Read the model definition and answer for the solid it produces. Units are mm, in the model's axes. Face numbers are marked on the shaded views. A direction names the side the tool comes from. Coordinates: 2 decimals unless noted, no trailing zeros. Loops run counter-clockwise (first coordinate to the right, second up) from the corner with the lowest first, then second, coordinate; pieces in that order, holes last.
Q1. Which of the six approach directions +Z, -Z, +X, -X, +Y, -Y give full straight-line access (tool end or side, diameter ignored) to the marked faces 1 and 2?
Q2. Flat-ended cylindrical pins translate along their axes: P1, Ø1.5, axis at x = 43.5, z = 3.5, coming from the -Y side; P2, Ø1.5, axis at y = 9, z = 2.5, coming from the -X side; P3, Ø2.5, axis at y = -28, z = 3, coming from the +X side; P4, Ø6, axis at x = 80.93, y = -12.5, coming from the +Z side. Find the tip coordinate at first contact, or state that the pin passes through.
Q3. Section D-D (x = 40) is taken. Give the vertices of the cut face in (y, z).
Q4. Straight lines are drawn through the part: line 1 (X direction, y = -26, z = 3.4); line 2 (X direction, y = -12.5, z = 0.9); line 3 (Y direction, x = 57, z = 3.6). For each, find the intervals that lie inside material, in ascending order.
Q5. Section C-C (x = -19) is taken. Give the vertices of the cut face in (y, z), then the cut area to 3 significant figures.
Q6. Section A-A (y = -28.5) is taken. Give the vertices of the cut face in (x, z).
Q7. Section B-B (z = 1.5) is taken. Give the vertices of the cut face in (x, y) (1 decimal).
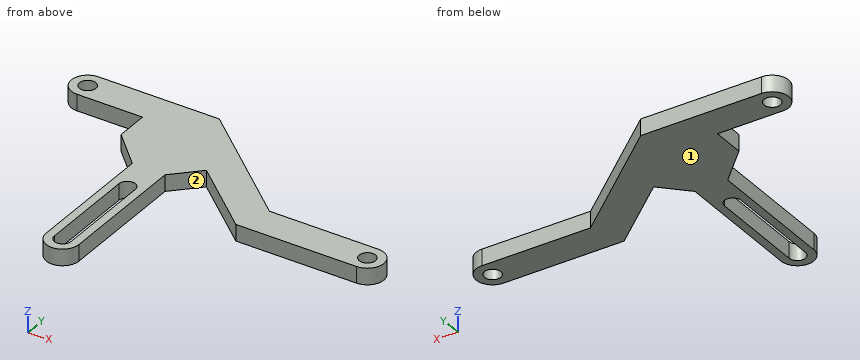
Autodesk Inventor part; units mm, degrees
ref_plane "YZ Plane" through (0, 0, 0) normal (1, 0, 0) x (0, 1, 0)
ref_plane "XZ Plane" through (0, 0, 0) normal (0, 1, 0) x (-1, 0, 0)
ref_plane "XY Plane" through (0, 0, 0) normal (0, 0, 1) x (1, 0, 0)
sketch "Sketch1" plane through (0, 0, 0) normal (0, 0, 1) x (1, 0, 0)
  line L0 (-24.0654, 17.5007) -> (10.9346, 17.5007) construction
  line L1 (45.9346, -12.4993) -> (80.9346, -12.4993) construction
  line L2 (10.9346, 17.5007) -> (45.9346, -12.4993) construction
  line L3 (-24.0654, 22.5007) -> (12.7842, 22.5007)
  line L4 (12.7842, 22.5007) -> (47.7842, -7.4993)
  line L5 (47.7842, -7.4993) -> (80.9346, -7.4993)
  line L6 (-24.0654, 12.5007) -> (-4.0654, 12.5007)
  line L7 (44.085, -17.4993) -> (80.9346, -17.4993)
  line L8 (10.9346, 17.5007) -> (10.9346, -47.4993) construction
  line L9 (15.9346, -7.4993) -> (15.9346, -47.4993)
  line L10 (22.4168, 1.0734) -> (44.085, -17.4993)
  arc A0 (-29.0654, 17.5007) -> (-24.0654, 12.5007) centre (-24.0654, 17.5007) ccw
  arc A1 (-24.0654, 22.5007) -> (-29.0654, 17.5007) centre (-24.0654, 17.5007) ccw
  arc A2 (85.9346, -12.4993) -> (80.9346, -7.4993) centre (80.9346, -12.4993) ccw
  arc A3 (80.9346, -17.4993) -> (85.9346, -12.4993) centre (80.9346, -12.4993) ccw
  arc A4 (10.9346, -52.4993) -> (15.9346, -47.4993) centre (10.9346, -47.4993) ccw
  arc A5 (5.9346, -47.4993) -> (10.9346, -52.4993) centre (10.9346, -47.4993) ccw
  line L11 (-4.0654, 12.5007) -> (-4.0654, 2.5007)
  line L12 (5.9346, -7.4993) -> (5.9346, -7.4993)
  line L13 (-4.0654, 2.5007) -> (5.9346, -7.4993)
  line L14 (15.9346, -7.4993) -> (23.5424, 0.1085)
  line L15 (5.9346, -47.4993) -> (5.9346, -7.4993)
  point P0 (0, 0)
  point P1 (-29.0654, 17.5007)
  point P2 (-4.0654, -7.4993)
  dimension "d0" = 35
  dimension "d4" = 35
  dimension "d5" = 35
  dimension "d6" = 30
  dimension "d7" = 5
  dimension "d8" = 5
  dimension "d10" = 5
  dimension "d11" = 5
  dimension "d13" = 65
  dimension "d14" = 5
  dimension "d15" = 5
  dimension "d16" = 5
  dimension "d34" = 5
  dimension "d35" = 5
  dimension "d36" = 5
  dimension "d37" = 5
  dimension "d41" = 20
  dimension "d43" = 10
  dimension "d44" = 10
  dimension "d47" = 135
extrude "Cuerpo" add sketch "Sketch1" along normal blind 5
sketch "Sketch2" plane through (0, 0, 5) normal (0, 0, 1) x (1, 0, 0)
  arc A0 (-24.0654, 22.5007) -> (-24.0654, 12.5007) centre (-24.0654, 17.5007) ccw
  arc A1 (80.9346, -17.4993) -> (80.9346, -7.4993) centre (80.9346, -12.4993) ccw
  point P0 (0, 0)
hole "Hole1" at (-24.0654, 17.5007, 5) at (80.9346, -12.4993, 5) direction (0, 0, -1) diameter 5 end through all
sketch "Sketch3" plane through (0, 0, 5) normal (0, 0, 1) x (1, 0, 0)
  arc A0 (5.9346, -47.4993) -> (15.9346, -47.4993) centre (10.9346, -47.4993) ccw construction
  line L0 (10.9346, -47.4993) -> (10.9346, -17.4993) construction
  line L1 (10.9346, -14.9993) -> (10.9346, -14.9993)
  line L2 (13.4346, -17.4993) -> (13.4346, -47.4993)
  line L3 (10.9346, -49.9993) -> (10.9346, -49.9993)
  line L4 (8.4346, -47.4993) -> (8.4346, -17.4993)
  arc A1 (10.9346, -14.9993) -> (8.4346, -17.4993) centre (10.9346, -17.4993) ccw
  arc A2 (13.4346, -17.4993) -> (10.9346, -14.9993) centre (10.9346, -17.4993) ccw
  arc A3 (8.4346, -47.4993) -> (10.9346, -49.9993) centre (10.9346, -47.4993) ccw
  arc A4 (10.9346, -49.9993) -> (13.4346, -47.4993) centre (10.9346, -47.4993) ccw
  point P0 (0, 0)
  point P1 (10.9346, -14.9993)
  point P2 (10.9346, -49.9993)
  dimension "d26" = 30
  dimension "d28" = 2.5
  dimension "d29" = 2.5
  dimension "d30" = 2.5
  dimension "d31" = 2.5
extrude "Ranura" cut sketch "Sketch3" against normal blind 5
sketch "Sketch4" plane through (0, 0, 5) normal (0, 0, 1) x (1, 0, 0)
  circle A0 centre (10.0854, 7.229) radius 12.5 construction
  point P0 (0, 0)
  dimension "d38" = 25
properties part number "BrazoV2" material "MDF Medium Density Fiberboard"
Numbers:
1. face 1: -Z, +X, -X, +Y, -Y
1. face 2: +Z, -Z, -Y
2. P1: stops at y = -17.5
2. P2: stops at x = -4.07
2. P3: stops at x = 15.93
2. P4: stops at z = 5
3. outline: (-14, 0) - (-0.83, 0) - (-0.83, 5) - (-14, 5) - close
4. line 1: x = 5.93 to 8.43, 13.43 to 15.93
4. line 2: x = 5.93 to 15.93, 38.25 to 78.43, 83.43 to 85.93
4. line 3: y = -17.5 to -7.5
5. outline: (12.5, 0) - (22.5, 0) - (22.5, 5) - (12.5, 5) - close
5. area: 50.0 mm2
6. outline: (5.93, 0) - (8.43, 0) - (8.43, 5) - (5.93, 5) - close; (13.43, 0) - (15.93, 0) - (15.93, 5) - (13.43, 5) - close
7. outline: (-24.1, 12.5) - (-4.1, 12.5) - (-4.1, 2.5) - (5.9, -7.5) - (5.9, -47.5) arc R5 ccw to (15.9, -47.5) - (15.9, -7.5) - (23.5, 0.1) - (44.1, -17.5) - (80.9, -17.5) arc R5 ccw to (80.9, -7.5) - (47.8, -7.5) - (12.8, 22.5) - (-24.1, 22.5) arc R5 ccw to start; hole circle Ø5 at (-24.1, 17.5); hole (8.4, -47.5) arc R2.5 ccw to (13.4, -47.5) - (13.4, -17.5) arc R2.5 ccw to (8.4, -17.5) - close; hole circle Ø5 at (80.9, -12.5)
